Input: part model. Units: mm. Frame: model coordinates. Face numbers are marked on the shaded views. A direction names the side the tool comes from. Round coordinates to 2 decimals unless told otherwise and drop trailing zeros. Loops run counter-clockwise (first coordinate to the right, second up) from the corner with the lowest first, then second, coordinate; pieces in that order, holes last. Notation, with made-up numbers: M 31,77.25 L 90,77.25 A18 cw 90,81.25 Z; hole C 68.25,28.5 d1. An arc over 180 degrees is marked long. Return JSON: item names as keys, results as strings. Group by question number.
1) Section D-D (z = 12.7). Output: boundary loops of the cut face in (x, y) (3 decimals), plus the area to 3 significant figures.
2) Material intervals for line 1 (X direction, y = 3.25, z = 5.08); line 2 (Y direction, x = 14, z = 7), sorted ascending. Write a range as from..to.
3) Section C-C (z = 23.5). Output: boundary loops of the cut face in (x, y) (3 decimals).
4) Section B-B (y = 11.75). Output: boundary loops of the cut face in (x, z), plus the area to 3 significant figures.
5) Mould query, pull axis Z, two halves, no side actions, for the marked faces 3, 4 and 5. Classes: +Z half, -Z half, draft (parallel to the pull), parting line (faces both ways), or undercut.
6) Contact query for flat-ended pins moving along their axis: P1, Ø10, axis at x = 14.5, z = 8, coming from the +Y side; P2, Ø11, axis at y = 11.303, z = 12.7, coming from the +X side; P3, Ø3, axis at y = 14, z = 3.5, coming from the +X side. Output: stop coordinate, or through.
7) Access query for the marked faces 1 and 2. Directions: +Z, -Z, +X, -X, +Y, -Y. A direction counts if a zero-diameter tool reaches every point of the face in a straight line with its end or side. Return the directions, or none.
8) Section A-A (z = 5.08). Output: boundary loops of the cut face in (x, y) (3 decimals).
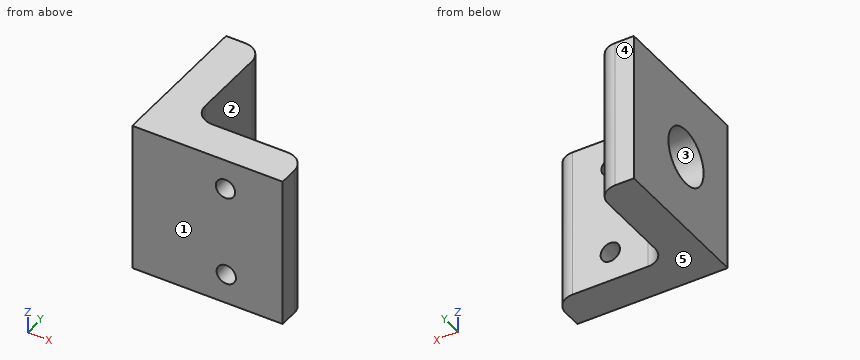
from build123d import *

# Parameters (mm, degrees)
BOSS_EXTRUDE1_DEPTH          = 25.4
F_4_CLEARANCE_HOLE1_D        = 3.2639
FILLET1_R                    = 3.175
F_3_8_0_374_DIAMETER_HOLE1_D = 9.4996


with BuildPart() as part:
    # Sketch1 → Boss-Extrude1 (new body)
    with BuildSketch(Plane.XY):
        Polygon((0, 25.4), (0, 0), (25.4, 0), (25.4, 6.35), (6.35, 6.35), (6.35, 25.4), align=None)
    extrude(amount=BOSS_EXTRUDE1_DEPTH)

    # #4 Clearance Hole1 (through all)
    with Locations(Plane(origin=(0, 6.35, 0), x_dir=(1, 0, 0), z_dir=(0, 1, 0))):
        with Locations((15.735159407, -20.32), (15.875, -5.08)):
            Hole(F_4_CLEARANCE_HOLE1_D / 2)

    # Fillet1
    fillet1_edges = [part.edges().sort_by_distance(p)[0] for p in [
        (6.35, 6.35, 12.7),
        (25.4, 6.35, 12.7),
        (6.35, 25.4, 12.7),
    ]]
    fillet(fillet1_edges, radius=FILLET1_R)

    # 3/8 (0.374) Diameter Hole1 (through all)
    with Locations(Plane(origin=(0, 0, 0), x_dir=(0, 0, -1), z_dir=(-1, 0, 0))):
        with Locations((-12.7, -11.303)):
            Hole(F_3_8_0_374_DIAMETER_HOLE1_D / 2)


solid = part.part
Returned:
{
 "1": {"outline": "M 0,0 L 25.4,0 L 25.4,3.175 A3.175 ccw 22.225,6.35 L 9.525,6.35 A3.175 cw 8.407,6.553 L 0,6.553 Z; M 0,16.053 L 6.35,16.053 L 6.35,22.225 A3.175 ccw 3.175,25.4 L 0,25.4 Z", "area": "218 mm^2"},
 "2": {"line 1": "x = 0..14.24, 17.51..25.4", "line 2": "y = 0..6.35"},
 "3": {"outline": "M 0,0 L 25.4,0 L 25.4,3.175 A3.175 ccw 22.225,6.35 L 9.525,6.35 A3.175 cw 6.35,9.525 L 6.35,22.225 A3.175 ccw 3.175,25.4 L 0,25.4 Z"},
 "4": {"outline": "M 0,0 L 6.35,0 L 6.35,7.97 L 0,7.97 Z; M 0,17.43 L 6.35,17.43 L 6.35,25.4 L 0,25.4 Z", "area": "101 mm^2"},
 "5": {"face 3": "undercut", "face 4": "draft", "face 5": "-Z half"},
 "6": {"P1": "stops at y = 6.35", "P2": "stops at x = 24.01", "P3": "stops at x = 6.35"},
 "7": {"face 1": "+Z, -Z, +X, -X, -Y", "face 2": "+Z, -Z, +X, +Y"},
 "8": {"outline": "M 0,0 L 14.243,0 L 14.243,6.35 L 9.525,6.35 A3.175 cw 6.35,9.525 L 6.35,22.225 A3.175 ccw 3.175,25.4 L 0,25.4 Z; M 17.507,0 L 25.4,0 L 25.4,3.175 A3.175 ccw 22.225,6.35 L 17.507,6.35 Z"}
}
